```python
from build123d import *

# Parameters (mm, degrees)
SKETCH1_W           = 20
SKETCH1_H           = 80
SKETCH1_R           = 2.5
BOSS_EXTRUDE1_DEPTH = 3
SKETCH2_W           = 20
SKETCH2_H           = 3
BOSS_EXTRUDE2_DEPTH = 20
SKETCH4_W           = 3.015323491
SKETCH4_H           = 23
BOSS_EXTRUDE4_DEPTH = 20
SKETCH7_R           = 2.5
CUT_EXTRUDE2_DEPTH  = 20


with BuildPart() as part:
    # Sketch1 → Boss-Extrude1 (new body)
    with BuildSketch(Plane(origin=(0, 0, 0), x_dir=(1, 0, 0), z_dir=(0, 1, 0))):
        Rectangle(SKETCH1_W, SKETCH1_H)
        with Locations((0, -30)):
            Circle(SKETCH1_R, mode=Mode.SUBTRACT)
        with Locations((0, 10)):
            Circle(SKETCH1_R, mode=Mode.SUBTRACT)
    extrude(amount=BOSS_EXTRUDE1_DEPTH)

    # Sketch2 → Boss-Extrude2 (add)
    with BuildSketch(Plane(origin=(0, 3, 0), x_dir=(1, 0, 0), z_dir=(0, 1, 0))):
        with Locations((0, 38.5)):
            Rectangle(SKETCH2_W, SKETCH2_H)
    extrude(amount=BOSS_EXTRUDE2_DEPTH)

    # Sketch4 → Boss-Extrude4 (add)
    with BuildSketch(Plane.ZY.offset(10)):
        with Locations((-38.492338254, 11.5)):
            Rectangle(SKETCH4_W, SKETCH4_H)
    extrude(amount=BOSS_EXTRUDE4_DEPTH)

    # Sketch7 → Cut-Extrude2 (cut)
    with BuildSketch(Plane(origin=(0, 0, -40), x_dir=(-1, 0, 0), z_dir=(0, 0, -1))):
        with Locations((16, 10)):
            Circle(SKETCH7_R)
    extrude(amount=-CUT_EXTRUDE2_DEPTH, mode=Mode.SUBTRACT)


solid = part.part
```
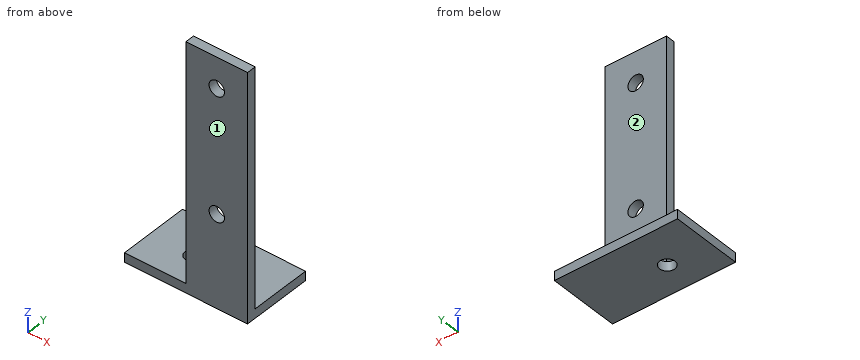
Verification items for the finished model (mm, model axes). Face numbers are marked on the shaded views. A direction names the side the tool comes from. Coordinates: 2 decimals unless noted, no trailing zeros. Loops run counter-clockwise (first coordinate to the right, second up) from the corner with the lowest first, then second, coordinate; pieces in that order, holes last. Notation, with made-up numbers: (22, 78) - (33, 78) arc R14 ccw to (33, 102) - close; hole circle Ø11 at (-37, -11.75). An arc over 180 degrees is marked (long way). Return JSON: item names as keys, results as strings.
1. Section check A-A, the plane z = 30. Record the boundary of the cut face in (x, y).
Established:
{"outline": "(-10, 0) - (-2.5, 0) - (-2.5, 3) - (-10, 3) - close; (2.5, 0) - (10, 0) - (10, 3) - (2.5, 3) - close"}
2. Section check D-D, the plane x = -16. Record the boundary of the cut face in (y, z), then the cut area to 3 significant figures.
Established:
{"outline": "(0, -40) - (7.5, -40) - (7.5, -36.98) - (0, -36.98) - close; (12.5, -40) - (23, -40) - (23, -36.98) - (12.5, -36.98) - close", "area": "54.3 mm2"}
3. Go/stop test with flat-tipped pins: pin 1 (5 mm diameter, centred on x = -1.5, y = 12, fed in from +Z); pin 2 (6.5 mm diameter, centred on x = 0, z = -10, fed in from +Y); pin 3 (1.5 mm diameter, centred on y = 1, z = 17.5, fed in from -X). Record where each tip stops, or that it passes through.
Established:
{"pin 1": "stops at z = -37", "pin 2": "stops at y = 3", "pin 3": "stops at x = -10"}
4. Thickness scan on L1, parallel to Z at x = 0, y = 1.9; L2, parallel to Y at x = -16, z = -39.2; L3, parallel to Z at x = -2, y = 1.75. Record the ranges inside material, lowest first.
Established:
{"L1": "z = -40 to -12.5, -7.5 to 27.5, 32.5 to 40", "L2": "y = 0 to 7.5, 12.5 to 23", "L3": "z = -40 to -11.5, -8.5 to 28.5, 31.5 to 40"}
5. Tool access check on the marked faces 1 and 2. Record the directions out of +Z, -Z, +X, -X, +Y, -Y that give a thin tool (end or side, any length) a straight path to the whole face; none if there is none.
Established:
{"face 1": "+Z, -Z, +X, -X, -Y", "face 2": "+Z, +X, -X, +Y"}
6. Section check C-C, the plane x = 0. Record the boundary of the cut face in (y, z), then the cut area to 3 significant figures.
Established:
{"outline": "(0, -40) - (23, -40) - (23, -37) - (3, -37) - (3, -12.5) - (0, -12.5) - close; (0, -7.5) - (3, -7.5) - (3, 27.5) - (0, 27.5) - close; (0, 32.5) - (3, 32.5) - (3, 40) - (0, 40) - close", "area": "270 mm2"}
